Design review of the part built by this model. Coordinates are the model's own, in mm. Face numbers are marked on the shaded views. A direction names the side the tool comes from. Coordinates: 2 decimals unless noted, no trailing zeros. Write each loop counter-clockwise with the first axis right and the second up, starting at its lowest first coordinate (ties: lowest second). Pieces come first, ordered by that corner, then holes. Notation, with made-up numbers: (-5.5, -1) -> (51.5, -1) arc R18 cw to (51.5, 3) -> close; hole circle Ø5 at (66, 35.25). An arc over 180 degrees is marked (long way). Return JSON: item names as keys, results as strings. Group by question number.
from build123d import *

# Parameters (mm, degrees)
SKETCH_1_R      = 6
EXTRUDE_1_DEPTH = 11


with BuildPart() as part:
    # 草图1 → 凸台-拉伸1 (new body)
    with BuildSketch(Plane.XY):
        with BuildLine():
            Line((-2.438629025, 12.259816005), (-1.560722576, 7.846282243))
            ThreePointArc((-1.560722576, 7.846282243), (-3.061467459, 7.39103626), (-4.444561864, 6.651756898))
            Line((-4.444561864, 6.651756898), (-6.944627913, 10.393370154))
            ThreePointArc((-6.944627913, 10.393370154), (-8.838834765, 8.838834765), (-10.393370154, 6.944627913))
            Line((-10.393370154, 6.944627913), (-6.651756898, 4.444561864))
            ThreePointArc((-6.651756898, 4.444561864), (-7.39103626, 3.061467459), (-7.846282243, 1.560722576))
            Line((-7.846282243, 1.560722576), (-12.259816005, 2.438629025))
            ThreePointArc((-12.259816005, 2.438629025), (-12.5, 0), (-12.259816005, -2.438629025))
            Line((-12.259816005, -2.438629025), (-7.846282243, -1.560722576))
            ThreePointArc((-7.846282243, -1.560722576), (-7.39103626, -3.061467459), (-6.651756898, -4.444561864))
            Line((-6.651756898, -4.444561864), (-10.393370154, -6.944627913))
            ThreePointArc((-10.393370154, -6.944627913), (-8.838834765, -8.838834765), (-6.944627913, -10.393370154))
            Line((-6.944627913, -10.393370154), (-4.444561864, -6.651756898))
            ThreePointArc((-4.444561864, -6.651756898), (-3.061467459, -7.39103626), (-1.560722576, -7.846282243))
            Line((-1.560722576, -7.846282243), (-2.438629025, -12.259816005))
            ThreePointArc((-2.438629025, -12.259816005), (0, -12.5), (2.438629025, -12.259816005))
            Line((2.438629025, -12.259816005), (1.560722576, -7.846282243))
            ThreePointArc((1.560722576, -7.846282243), (3.061467459, -7.39103626), (4.444561864, -6.651756898))
            Line((4.444561864, -6.651756898), (6.944627913, -10.393370154))
            ThreePointArc((6.944627913, -10.393370154), (8.838834765, -8.838834765), (10.393370154, -6.944627913))
            Line((10.393370154, -6.944627913), (6.651756898, -4.444561864))
            ThreePointArc((6.651756898, -4.444561864), (7.39103626, -3.061467459), (7.846282243, -1.560722576))
            Line((7.846282243, -1.560722576), (12.259816005, -2.438629025))
            ThreePointArc((12.259816005, -2.438629025), (12.5, 0), (12.259816005, 2.438629025))
            Line((12.259816005, 2.438629025), (7.846282243, 1.560722576))
            ThreePointArc((7.846282243, 1.560722576), (7.39103626, 3.061467459), (6.651756898, 4.444561864))
            Line((6.651756898, 4.444561864), (10.393370154, 6.944627913))
            ThreePointArc((10.393370154, 6.944627913), (8.838834765, 8.838834765), (6.944627913, 10.393370154))
            Line((6.944627913, 10.393370154), (4.444561864, 6.651756898))
            ThreePointArc((4.444561864, 6.651756898), (3.061467459, 7.39103626), (1.560722576, 7.846282243))
            Line((1.560722576, 7.846282243), (2.438629025, 12.259816005))
            ThreePointArc((2.438629025, 12.259816005), (0, 12.5), (-2.438629025, 12.259816005))
        make_face()
        Circle(SKETCH_1_R, mode=Mode.SUBTRACT)
    extrude(amount=EXTRUDE_1_DEPTH)


solid = part.part
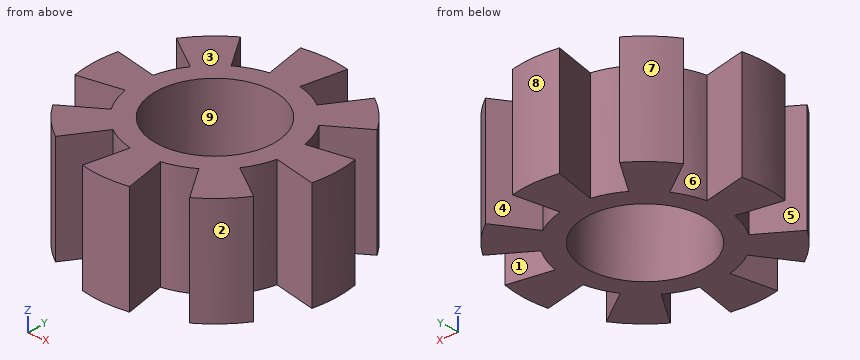
Q1. Wall thickness on L1, parallel to Y at x = 0, z = 3; L2, parallel to Y at x = 9, z = 4.25; L3, parallel to Y at x = -5.25, z = 1.5: over which ranges is each line inside the solid? List them lowest first.
Q2. For P1, Ø6, axis at x = 6.5, z = 8, coming from the +Y side; P2, Ø5, axis at x = -6.5, z = 7, coming from the -Y side; P3, Ø5, axis at x = 3, z = 2, coming from the +Y side, all flat-tipped, find the tip position at first contact; note any pin that passes through.
Q3. For the marked faces 1, 2, 3, 4 and 5, list the 3-axis set-ups (+Z, -Z, +X, -X, +Y, -Y) from which the entire face can be reached by the end or side of a thin tool; tool diameter is ignored.
Q4. We need section B-B on x = 0. Write out the cut boundary in (y, z), plus the area to 3 significant figures.
Q5. We need section D-D on x = -7.5. Write out the cut boundary in (y, z), plus the area to 3 significant figures.
Q6. The part is to be moulded in two halves that separate along X. For the marked faces 6, 7, 8 and 9, say which applies: +X half, -X half, draft (parallel to the pull), parting line (faces both ways), or undercut.
Findings below:
{
 "1": {"L1": "y = -12.5 to -6, 6 to 12.5", "L2": "y = -8.67 to -6.01, -1.79 to 1.79, 6.01 to 8.67", "L3": "y = -7.86 to -2.9, 2.9 to 7.86"},
 "2": {"P1": "stops at y = 10.39", "P2": "stops at y = -10.39", "P3": "stops at y = 12.49"},
 "3": {"face 1": "+Z, -Z", "face 2": "+Z, -Z, +X, -Y", "face 3": "+Z, +X, -X, +Y, -Y", "face 4": "+Z, -Z, +Y", "face 5": "+Z, -Z, -X"},
 "4": {"outline": "(-12.5, 0) -> (-6, 0) -> (-6, 11) -> (-12.5, 11) -> close; (6, 0) -> (12.5, 0) -> (12.5, 11) -> (6, 11) -> close", "area": "143 mm^2"},
 "5": {"outline": "(-10, 0) -> (-5.01, 0) -> (-5.01, 11) -> (-10, 11) -> close; (-2.78, 0) -> (2.78, 0) -> (2.78, 11) -> (-2.78, 11) -> close; (5.01, 0) -> (10, 0) -> (10, 11) -> (5.01, 11) -> close", "area": "171 mm^2"},
 "6": {"face 6": "undercut", "face 7": "-X half", "face 8": "parting line", "face 9": "undercut"}
}
